```python
from build123d import *

# Parameters (mm, degrees)
F0_W     = 205
F0_H     = 230
F1_DEPTH = 15
F2_W     = 200.2
F2_H     = 225.2
F3_DEPTH = 13.8
F4_W     = 200.2
F4_H     = 225.2
F5_DEPTH = 9.99
F7_DEPTH = 9.99
F9_DEPTH = 9.99


with BuildPart() as f1:
    # F0 (on Top) → F1 (new body)
    with BuildSketch(Plane.XY):
        with Locations((102.5, 115)):
            Rectangle(F0_W, F0_H)
    extrude(amount=F1_DEPTH)

    # F2 (on face) → F3 (cut, through all)
    with BuildSketch(Plane.XY.offset(15)):
        with Locations((102.5, 115)):
            Rectangle(F2_W, F2_H)
    extrude(amount=-F3_DEPTH, mode=Mode.SUBTRACT)

    # F4 (on face) → F5 (join, through all)
    with BuildSketch(Plane.XY.offset(1.2)):
        with Locations((102.5, 115)):
            Rectangle(F4_W, F4_H)
        Polygon((4.8, 149), (4.8, 225.2), (101.9, 225.2), (103.1, 225.2), (200.2, 225.2), (200.2, 149), (200.2, 147.8), (200.2, 4.8), (103.1, 4.8), (101.9, 4.8), (4.8, 4.8), (4.8, 147.8), align=None, mode=Mode.SUBTRACT)
        Polygon((103.1, 225.2), (101.9, 225.2), (101.9, 149), (4.8, 149), (4.8, 147.8), (101.9, 147.8), (101.9, 4.8), (103.1, 4.8), (103.1, 147.8), (200.2, 147.8), (200.2, 149), (103.1, 149), align=None)
    extrude(amount=F5_DEPTH)

    # F6 (on face) → F7 (cut, through all)
    with BuildSketch(Plane.XY.offset(11.19)):
        with BuildLine():
            Line((103.1, 154.7215899899), (103.1, 149))
            Line((103.1, 149), (108.8215899899, 149))
            ThreePointArc((108.8215899899, 149), (106.9901280605, 152.8901280605), (103.1, 154.7215899899))
        make_face()
        with BuildLine():
            Line((102.5, 148.4), (103.1, 149))
            Line((103.1, 149), (103.1, 154.7215899899))
            ThreePointArc((103.1, 154.7215899899), (102.5, 154.75), (101.9, 154.7215899899))
            Line((101.9, 154.7215899899), (101.9, 149))
            Line((101.9, 149), (102.5, 148.4))
        make_face()
        with BuildLine():
            Line((96.1784100101, 149), (101.9, 149))
            Line((101.9, 149), (101.9, 154.7215899899))
            ThreePointArc((101.9, 154.7215899899), (98.0098719395, 152.8901280605), (96.1784100101, 149))
        make_face()
        with BuildLine():
            Line((96.1784100101, 147.8), (101.9, 147.8))
            Line((101.9, 147.8), (101.9, 149))
            Line((101.9, 149), (96.1784100101, 149))
            ThreePointArc((96.1784100101, 149), (96.15, 148.4), (96.1784100101, 147.8))
        make_face()
        Polygon((101.9, 147.8), (102.5, 148.4), (101.9, 149), align=None)
        with BuildLine():
            Line((108.8215899899, 149), (103.1, 149))
            Line((103.1, 149), (102.5, 148.4))
            Line((102.5, 148.4), (103.1, 147.8))
            Line((103.1, 147.8), (108.8215899899, 147.8))
            ThreePointArc((108.8215899899, 147.8), (108.8428935209, 148.0996638847), (108.85, 148.4))
            ThreePointArc((108.85, 148.4), (108.8428935209, 148.7003361153), (108.8215899899, 149))
        make_face()
        with BuildLine():
            Line((103.1, 147.8), (102.5, 148.4))
            Line((102.5, 148.4), (101.9, 147.8))
            Line((101.9, 147.8), (101.9, 142.0784100101))
            ThreePointArc((101.9, 142.0784100101), (102.5, 142.05), (103.1, 142.0784100101))
            Line((103.1, 142.0784100101), (103.1, 147.8))
        make_face()
        with BuildLine():
            Line((108.8215899899, 147.8), (103.1, 147.8))
            Line((103.1, 147.8), (103.1, 142.0784100101))
            ThreePointArc((103.1, 142.0784100101), (106.9901280605, 143.9098719395), (108.8215899899, 147.8))
        make_face()
        with BuildLine():
            Line((101.9, 142.0784100101), (101.9, 147.8))
            Line((101.9, 147.8), (96.1784100101, 147.8))
            ThreePointArc((96.1784100101, 147.8), (98.0098719395, 143.9098719395), (101.9, 142.0784100101))
        make_face()
    extrude(amount=-F7_DEPTH, mode=Mode.SUBTRACT)

    # F8 (on face) → F9 (join, through all)
    with BuildSketch(Plane.XY.offset(1.2)):
        Polygon((200.2, 44.139730379), (103.1, 18.9472891124), (103.1, 17.7075587334), (200.2, 42.9), align=None)
        Polygon((101.9, 18.6359510123), (48.5716691298, 4.8), (53.35, 4.8), (101.9, 17.3962206333), align=None)
    extrude(amount=F9_DEPTH)


solid = f1.part
```
Work out the finished part from the listing and answer in its coordinate system (mm). A direction names the side the tool comes from. Round coordinates to 2 decimals unless told otherwise and drop trailing zeros. Loops run counter-clockwise (first coordinate to the right, second up) from the corner with the lowest first, then second, coordinate; pieces in that order, holes last.
(1) The mould has two halves that part along Y. Classify faces 3 (the flat face through (88, 8, 1.2)), 4 (the flat face through (0, 113, 7)), 5 (the flat face through (101, 230, 7)), 6 (the flat face through (101, 0, 7)): pulls with the +Y half, pulls with the -Y half, needs draft (parallel to the pull), parting line crosses it, or undercut.
Computed values:
face 3: undercut
face 4: needs draft
face 5: pulls with the +Y half
face 6: pulls with the -Y half
(2) Find the intervals of material crossed by L1, parallel to X at y = 209, z = 7.25; L2, parallel to Y at x = 25, z = 11; L3, parallel to Y at x = 96, z = 13, in increasing order.
Computed values:
L1: x = 0 to 4.8, 101.9 to 103.1, 200.2 to 205
L2: y = 0 to 4.8, 147.8 to 149, 225.2 to 230
L3: y = 0 to 2.4, 227.6 to 230
(3) The part is cut by section D-D, the plane y = 65. Give the vertices of the cut face in (x, z).
Computed values:
outline: (0, 0) - (205, 0) - (205, 15) - (202.6, 15) - (202.6, 11.19) - (200.2, 11.19) - (200.2, 1.2) - (103.1, 1.2) - (103.1, 11.19) - (101.9, 11.19) - (101.9, 1.2) - (4.8, 1.2) - (4.8, 11.19) - (2.4, 11.19) - (2.4, 15) - (0, 15) - close
(4) For faces 1 (the flat face through (103.1, 11, 6)), 2 (the flat face through (101, 117, 0)), determine the directions among +Z, -Z, +X, -X, +Y, -Y from which every point of the face is accessible in a straight line to the end or side of a thin tool.
Computed values:
face 1: +Z
face 2: -Z, +X, -X, +Y, -Y
(5) The part is cut by section B-B, the plane y = 145. Give the vertices of the cut face in (x, z).
Computed values:
outline: (0, 0) - (205, 0) - (205, 15) - (202.6, 15) - (202.6, 11.19) - (200.2, 11.19) - (200.2, 1.2) - (4.8, 1.2) - (4.8, 11.19) - (2.4, 11.19) - (2.4, 15) - (0, 15) - close
(6) The part is cut by section A-A, the plane z = 6.5. Give the number of separate pieces and of enclosed holes in the cut face, and give its area (3 significant figures).
Computed values:
separate pieces: 1
enclosed holes: 3
area: 4,740 mm2
(7) The part is cut by section C-C, the plane x = 13. Give the vertices of the cut face in (y, z), and give its area (3 significant figures).
Computed values:
outline: (0, 0) - (230, 0) - (230, 15) - (227.6, 15) - (227.6, 11.19) - (225.2, 11.19) - (225.2, 1.2) - (149, 1.2) - (149, 11.19) - (147.8, 11.19) - (147.8, 1.2) - (4.8, 1.2) - (4.8, 11.19) - (2.4, 11.19) - (2.4, 15) - (0, 15) - close
area: 402 mm2
